Work out the finished part from the listing and answer in its coordinate system (mm). A direction names the side the tool comes from. Round coordinates to 2 decimals unless told otherwise and drop trailing zeros. Order: outer loops, then holes, each group sorted by start corner. A loop starts at its lowest first (then second) coordinate and runs counter-clockwise, first axis right, second up.
from build123d import *

# Parameters (mm, degrees)
SKETCH1_W           = 44
SKETCH1_H           = 20
BOSS_EXTRUDE1_DEPTH = 5
SKETCH2_W           = 5
SKETCH2_H           = 20
SKETCH2_W_2         = 10
BOSS_EXTRUDE2_DEPTH = 10
CUT_EXTRUDE1_REACH  = 51.356
SKETCH4_R           = 1.75
SKETCH5_R           = 1.5
CUT_EXTRUDE2_DEPTH  = 7
FILLET1_R           = 1


with BuildPart() as part:
    # Sketch1 → Boss-Extrude1 (new body)
    with BuildSketch(Plane.XY):
        with Locations((22, 10)):
            Rectangle(SKETCH1_W, SKETCH1_H)
    extrude(amount=BOSS_EXTRUDE1_DEPTH)

    # Sketch2 → Boss-Extrude2 (add)
    with BuildSketch(Plane.XY.offset(5)):
        with Locations((2.5, 10)):
            Rectangle(SKETCH2_W, SKETCH2_H)
        with Locations((22, 10)):
            Rectangle(SKETCH2_W_2, SKETCH2_H)
        with Locations((41.5, 10)):
            Rectangle(SKETCH2_W, SKETCH2_H)
    extrude(amount=BOSS_EXTRUDE2_DEPTH)

    # Sketch4 → Cut-Extrude1 (cut, up to next)
    with BuildSketch(Plane.XY.offset(5), mode=Mode.PRIVATE) as cut_extrude1_sk1:
        with Locations((11, 10)):
            Circle(SKETCH4_R)
    cut_extrude1_tool1 = extrude(cut_extrude1_sk1.sketch, amount=-CUT_EXTRUDE1_REACH, mode=Mode.PRIVATE) & part.part
    # Sketch4 → Cut-Extrude1 (cut, up to next)
    with BuildSketch(Plane.XY.offset(5), mode=Mode.PRIVATE) as cut_extrude1_sk2:
        with Locations((33, 10)):
            Circle(SKETCH4_R)
    cut_extrude1_tool2 = extrude(cut_extrude1_sk2.sketch, amount=-CUT_EXTRUDE1_REACH, mode=Mode.PRIVATE) & part.part
    add(cut_extrude1_tool1.solids().sort_by_distance((11, 10, 5))[0], mode=Mode.SUBTRACT)
    add(cut_extrude1_tool2.solids().sort_by_distance((33, 10, 5))[0], mode=Mode.SUBTRACT)

    # Sketch5 → Cut-Extrude2 (cut)
    with BuildSketch(Plane.XY.offset(15)):
        with Locations((22, 15)):
            Circle(SKETCH5_R)
        with Locations((22, 5)):
            Circle(SKETCH5_R)
    extrude(amount=-CUT_EXTRUDE2_DEPTH, mode=Mode.SUBTRACT)

    # Fillet1
    fillet1_edges = [part.edges().sort_by_distance(p)[0] for p in [
        (11, 0, 5),
        (5, 10, 5),
        (5, 0, 10),
        (5, 20, 10),
        (33, 0, 5),
        (11, 20, 5),
        (17, 10, 5),
        (17, 20, 10),
        (17, 0, 10),
        (27, 10, 5),
        (27, 0, 10),
        (27, 20, 10),
        (17, 10, 15),
        (27, 10, 15),
        (33, 20, 5),
        (39, 0, 10),
        (39, 10, 5),
        (39, 20, 10),
        (0, 20, 7.5),
        (44, 20, 7.5),
        (44, 0, 7.5),
        (0, 0, 7.5),
    ]]
    fillet(fillet1_edges, radius=FILLET1_R)


solid = part.part
Item 1: Find section D-D (z = 7.5). Write down the section's boundary in (x, y).
Item 2: A tool of negligible diameter and unlimited length cuts with its end or side. For faces 4 (the face through (17.301, 0.285, 10.563)), 5 (the face through (17, 10, 10)), 6 (the face through (4.699, 19.715, 10.563)), 7 (the face through (2, 10, 15)), from which of +Z, -Z, +X, -X, +Y, -Y can it reach the whole face along a straight path? Write none if from no direction.
Item 3: Given pin 1 (3 mm diameter, centred on x = 33.5, y = 5.5, fed in from +Z); pin 2 (3 mm diameter, centred on x = 7, y = 8.5, fed in from +Z), each flat-ended and moving along its own axis, determine where each tip first touches the part or whether it passes through.
Item 4: Find the intervals of material crossed by line 1 along Y through (x, z) = (22, 13); line 2 along X through (y, z) = (10, 13.5); line 3 along Y through (x, z) = (11, 3), in increasing order.
Item 5: Find section B-B (x = 33). Write down the section's boundary in (y, z).
Item 6: Find section C-C (y = 10). Write down the section's boundary in (x, z).
Item 7: Find section A-A (z = 10.25). Write down the section's boundary in (x, y), plus the area to 3 significant figures.
Item 8: For a pull along X with two mould halves and no side action, classify faces 1 (the face through (0.285, 0.301, 7.605)), 2 (the face through (11.9, 11.5, 2.5)), 3 (the face through (41, 10, 15)) as released by +X, released by -X, zero draft, split by the parting line, or undercut.
Model answer:
1. outline: (0, 1) arc R1 ccw to (1, 0) - (4, 0) arc R1 ccw to (5, 1) - (5, 19) arc R1 ccw to (4, 20) - (1, 20) arc R1 ccw to (0, 19) - close; (17, 1) arc R1 ccw to (18, 0) - (26, 0) arc R1 ccw to (27, 1) - (27, 19) arc R1 ccw to (26, 20) - (18, 20) arc R1 ccw to (17, 19) - close; (39, 1) arc R1 ccw to (40, 0) - (43, 0) arc R1 ccw to (44, 1) - (44, 19) arc R1 ccw to (43, 20) - (40, 20) arc R1 ccw to (39, 19) - close
2. face 4: +Z, -Y
2. face 5: +Z, +Y, -Y
2. face 6: +Z, +Y
2. face 7: +Z, +X, -X, +Y, -Y
3. pin 1: stops at z = 5
3. pin 2: stops at z = 5.13
4. line 1: y = 0 to 3.5, 6.5 to 13.5, 16.5 to 20
4. line 2: x = 0 to 5, 17 to 27, 39 to 44
4. line 3: y = 0 to 8.25, 11.75 to 20
5. outline: (0, 0) - (8.25, 0) - (8.25, 5) - (1, 5) arc R1 ccw to (0, 4) - close; (11.75, 0) - (20, 0) - (20, 4) arc R1 ccw to (19, 5) - (11.75, 5) - close
6. outline: (0, 0) - (9.25, 0) - (9.25, 5) - (6, 5) arc R1 cw to (5, 6) - (5, 15) - (0, 15) - close; (12.75, 0) - (31.25, 0) - (31.25, 5) - (28, 5) arc R1 cw to (27, 6) - (27, 14) arc R1 ccw to (26, 15) - (18, 15) arc R1 ccw to (17, 14) - (17, 6) arc R1 cw to (16, 5) - (12.75, 5) - close; (34.75, 0) - (44, 0) - (44, 15) - (39, 15) - (39, 6) arc R1 cw to (38, 5) - (34.75, 5) - close
7. outline: (0, 1) arc R1 ccw to (1, 0) - (4, 0) arc R1 ccw to (5, 1) - (5, 19) arc R1 ccw to (4, 20) - (1, 20) arc R1 ccw to (0, 19) - close; (17, 1) arc R1 ccw to (18, 0) - (26, 0) arc R1 ccw to (27, 1) - (27, 19) arc R1 ccw to (26, 20) - (18, 20) arc R1 ccw to (17, 19) - close; (39, 1) arc R1 ccw to (40, 0) - (43, 0) arc R1 ccw to (44, 1) - (44, 19) arc R1 ccw to (43, 20) - (40, 20) arc R1 ccw to (39, 19) - close; hole circle Ø3 at (22, 5); hole circle Ø3 at (22, 15)
7. area: 383 mm2
8. face 1: released by -X
8. face 2: undercut
8. face 3: zero draft
